from build123d import *

# Parameters (mm, degrees)
CUT_EXTRUDE_1_DEPTH      = 10
PATTERN_CIRCULAR_1_COUNT = 3
FILLET_1_R               = 0.5
SCALE_1_SCALE            = 0.5


with BuildPart() as part:
    # Эскиз1 → Повернуть1 (revolve)
    with BuildSketch(Plane(origin=(0, 0, 0), x_dir=(0, 0, -1), z_dir=(1, 0, 0)), mode=Mode.PRIVATE) as revolve_1_sk:
        Polygon((-9, 0), (-9, 2), (1, 2), (1, 5), (3, 5), (3.7, 5.5), (8.916460066, 17.5), (23.4, 17.5), (23.4, 16), (9.9, 16), (7.009211714, 9.35), (7.009211714, 5), (9, 5), (9, 0), align=None)
    revolve(revolve_1_sk.sketch.rotate(Axis((0, 0, -9), (0, 0, -1)), 90), axis=Axis((0, 0, -9), (0, 0, -1)))

    # Эскиз2 → Вырез-Вытянуть1 (cut)
    with BuildSketch(Plane.XY.offset(-1)):
        with BuildLine():
            Line((1.55, 14.5641447), (-1.55, 14.5641447))
            ThreePointArc((-1.55, 14.5641447), (-6.235, 9.8791447), (-1.55, 5.1941447))
            Line((-1.55, 5.1941447), (1.55, 5.1941447))
            ThreePointArc((1.55, 5.1941447), (6.235, 9.8791447), (1.55, 14.5641447))
        make_face()
    cut_extrude_1 = extrude(amount=-CUT_EXTRUDE_1_DEPTH, mode=Mode.SUBTRACT)

    # Круговой массив1: Вырез-Вытянуть1 ×3 about axis
    pattern_circular_1_axis = Axis((0, 0, 0), (0, 0, 1))
    for i in range(1, PATTERN_CIRCULAR_1_COUNT):
        add(cut_extrude_1.rotate(pattern_circular_1_axis, i * 360 / PATTERN_CIRCULAR_1_COUNT), mode=Mode.SUBTRACT)

    # Скругление1
    fillet_1_edges = [part.edges().sort_by_distance(p)[0] for p in [
        (-17.5, 0, -23.4),
        (-17.5, 0, -8.916460066),
        (-5, 0, -1),
    ]]
    fillet(fillet_1_edges, radius=FILLET_1_R)


with BuildPart() as part_1:
    # Масштаб1: scaled about (3.2e-07, -3.26e-07, -11.771980124)
    add(part.part.scale(SCALE_1_SCALE).moved(Location((1.6e-07, -1.63e-07, -5.885990062))))


solid = part_1.part
Verification items for the finished model (mm, model axes). A direction names the side the tool comes from. Coordinates: 2 decimals unless noted, no trailing zeros. Loops run counter-clockwise (first coordinate to the right, second up) from the corner with the lowest first, then second, coordinate; pieces in that order, holes last. Notation, with made-up numbers: (47, -2) -> (93, -2) arc R23 ccw to (93, 27) -> close; hole circle Ø11 at (81.25, 0). An arc over 180 degrees is marked (long way). Answer as CSV lines item,"result".
1) Depth check by flat-ended pin: pin 1 (3 mm diameter, centred on x = -1.5, y = -5.5, fed in from +Z); pin 2 (1.5 mm diameter, centred on x = -1, y = 0.5, fed in from -Z); pin 3 (8 mm diameter, centred on y = 6, z = -10, fed in from +X). Enter the tip coordinate at first touch or a pass-through.
Found:
pin 1,"stops at z = -8.37"
pin 2,"stops at z = -10.39"
pin 3,"stops at x = 8.51"
2) Release check for a two-part mould opening along X. For faces 1 (the flat face through (-6.312, -3.632, -10.118)), 2 (the cylindrical face through (1, 0, -4)), 3 (the flat face through (0, 0, -1.386)) record: +X half, -X half, draft (parallel to the pull), parting line (faces both ways), or undercut.
Found:
face 1,"undercut"
face 2,"parting line"
face 3,"draft"
3) Cross-section at B-B, the plane z = -8.25. Record the cut outline in (x, y) (1 decimal).
Found:
outline,"(-3.9, 0.4) arc R2.3 cw to (-2.6, -0.6) -> (-1.9, -2) arc R2.3 cw to (-1.6, -3.6) arc R3.9 ccw to (1.6, -3.6) arc R2.3 cw to (1.9, -2) -> (2.6, -0.6) arc R2.3 cw to (3.9, 0.4) arc R3.9 ccw to (2.3, 3.2) arc R2.3 cw to (0.8, 2.6) -> (-0.8, 2.6) arc R2.3 cw to (-2.3, 3.2) arc R3.9 ccw to start"
4) Thickness scan on L1, parallel to X at y = 0, z = -15.5; L2, parallel to X at y = -2.75, z = -13. Record the ranges inside material, lowest first. Write a range as from..to.
Found:
L1,"x = -8.75..-8, 8..8.75"
L2,"x = -8.31..-7.51, 7.51..8.31"
5) Tool access check on faces 4 (the flat face through (-1, -1, -6.386)), 5 (the cylindrical face through (-3.06, 4.42, -9.43)), 6 (the flat face through (0, 0, -10.386)). Record the directions out of +Z, -Z, +X, -X, +Y, -Y that give a thin tool (end or side, any length) a straight path to the whole face; none if there is none.
Found:
face 4,"+Z"
face 5,"+Z, -Z"
face 6,"-Z"
6) Cross-section at A-A, the plane z = -11.25. Record the cut outline in (x, y), then the cut area to 3 significant figures.
Found:
outline,"circle Ø17.5 at (0, 0); hole circle Ø16 at (0, 0)"
area,"39.5 mm2"
